Answer from the drawing. Dimensions are ordinates in mm from the lowest x, y and z of the part. A direction names the side the tool comes from. Give positions to 0.01 mm unless a question says otherwise; leave off trailing zeros. Order: outer loops, then holes, each group sorted by start corner. A loop starts at its lowest first (then second) coordinate and runs counter-clockwise, first axis right, second up. Notation, with made-up numbers: (8.5, -17.75) - (24.5, -17.75) arc R22 cw to (24.5, 17.25) - close; hole circle Ø6 at (-40, -28.5). An arc over 180 degrees is marked (long way). One line per item, written item: value. Start each with the question number.
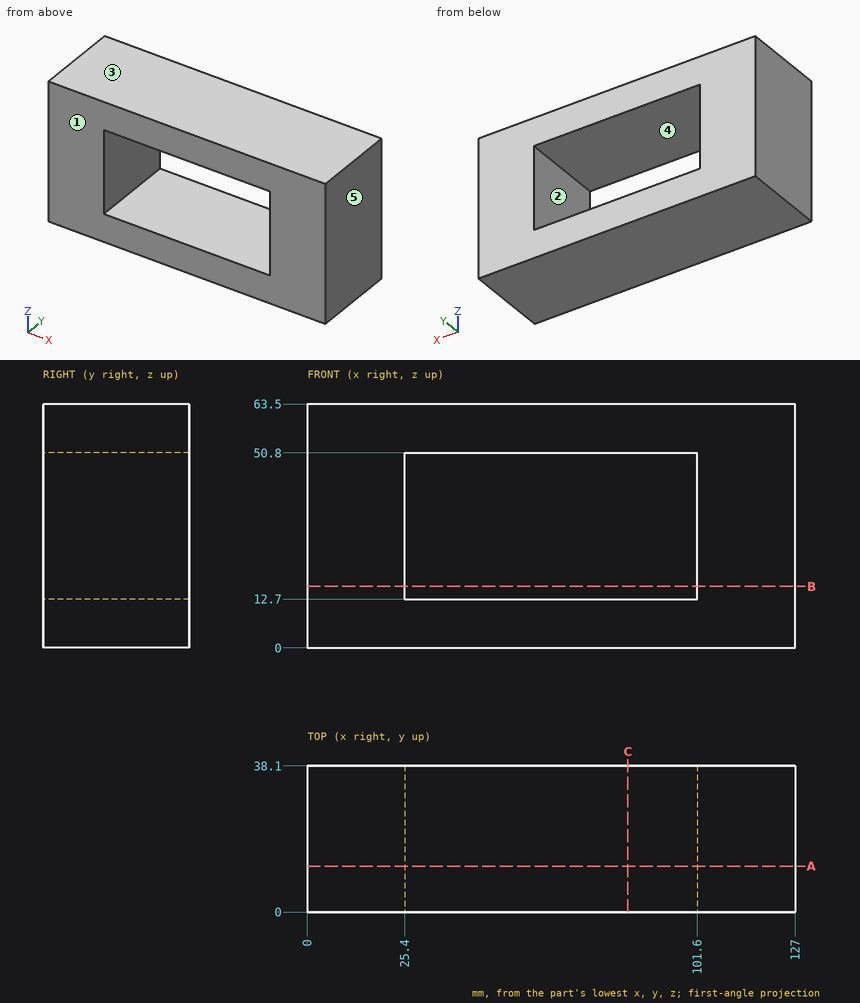
1) Section C-C on x = 83.5 is taken. Write down the section's boundary in (y, z).
2) Section B-B on z = 16 is taken. Write down the section's boundary in (x, y), plus the area to 3 significant figures.
3) The mould has two halves that part along X. Classify the marked faces 3, 4 and 5: +X half, -X half, draft (parallel to the pull), parting line (faces both ways), or undercut.
4) Section A-A on y = 12 is taken. Write down the section's boundary in (x, z).
5) Find the intervals of material crossed by probe 1 along X at (y, z) = (20, 38); probe 2 along Z at (x, y) = (80.5, 10.5), in increasing order. Write a range as from..to.
6) For the marked faces 1 and 2, determine the directions among +Z, -Z, +X, -X, +Y, -Y from which every point of the face is accessible in a straight line to the end or side of a thin tool.
Solved:
1. outline: (0, 0) - (38.1, 0) - (38.1, 12.7) - (0, 12.7) - close; (0, 50.8) - (38.1, 50.8) - (38.1, 63.5) - (0, 63.5) - close
2. outline: (0, 0) - (25.4, 0) - (25.4, 38.1) - (0, 38.1) - close; (101.6, 0) - (127, 0) - (127, 38.1) - (101.6, 38.1) - close
2. area: 1,940 mm2
3. face 3: draft
3. face 4: undercut
3. face 5: +X half
4. outline: (0, 0) - (127, 0) - (127, 63.5) - (0, 63.5) - close; hole (25.4, 12.7) - (101.6, 12.7) - (101.6, 50.8) - (25.4, 50.8) - close
5. probe 1: x = 0..25.4, 101.6..127
5. probe 2: z = 0..12.7, 50.8..63.5
6. face 1: +Z, -Z, +X, -X, -Y
6. face 2: +Y, -Y
